Build history of the part. All positions in model axes, mm. A direction names the side the tool comes from. Coordinates: 2 decimals unless noted, no trailing zeros. Write each loop counter-clockwise with the first axis right and the second up, starting at its lowest first coordinate (ties: lowest second). Pieces come first, ordered by that corner, then holes. Notation, with made-up numbers: (15, 19) -> (70, 19) arc R29 ccw to (70, 48) -> close; hole circle Ø10 at (-4.75, -34). An arc over 180 degrees is marked (long way). Write each question's results on one line, items separated by ' | '. Start each with the question number.
Q1. Tool access for faces 1 (the face through (84, 57, 0)), 2 (the face through (-63, -41, 2.9)), 3 (the face through (23, -13, -3)), 4 (the face through (21.48, 18.41, 3.83)): list every direction of +Z, -Z, +X, -X, +Y, -Y with a clear straight run to the whole face (end or side of a thin tool).
Q2. Drop flat-ended pins along their axis: pin 1 Ø13.5 at (x, y) = (89.5, -24) entering from -Z; pin 2 Ø8.5 at (x, y) = (11, 34.5) entering from -Z. Give the stop position or say it passes through.
Q3. Drill centre lines: line 1 (X direction, y = 60, z = -0.5); line 2 (X direction, y = 15, z = 0.5); line 3 (Z direction, x = -38.5, y = -1). Where is each one in solid material? Low to high.
Q4. Saw through at C-C on x = 81. Give the cut face in (y, z), and give its area (3 significant figures).
Q5. Two-plate mould, pull along X, no slides. Class faces 5 (the face through (-37, 45, -3)), 6 (the face through (11.09, 35.17, 3.83)), 7 (the face through (52.7, -27.8, -3)): released by +X, released by -X, zero draft, split by the parting line, or undercut.
Q6. Saw through at A-A on y = -2. Give the cut face in (x, z), and give its area (3 significant figures).
from build123d import *

# Parameters (mm, degrees)
SKETCH_1_W           = 180
SKETCH_1_H           = 108
EXTRUDE_4_DEPTH      = 6
SKETCH_3_R           = 2.85
EXTRUDE_8_DEPTH      = 5.7
SKETCH_4_R           = 2.85
EXTRUDE_9_DEPTH      = 3.1
SKETCH_5_R           = 2.85
CUT_EXTRUDE_1_DEPTH  = 3.1
SKETCH_7_R           = 2.85
CUT_EXTRUDE_2_DEPTH  = 3.1
SKETCH_8_R           = 2.85
CUT_EXTRUDE_3_DEPTH  = 3.1
SKETCH_9_R           = 2.85
CUT_EXTRUDE_4_DEPTH  = 3.1
SKETCH_10_R          = 1.51
CUT_EXTRUDE_5_DEPTH  = 3.1
SKETCH_11_R          = 1.51
CUT_EXTRUDE_6_DEPTH  = 3.1
SKETCH_12_R          = 1.51
CUT_EXTRUDE_7_DEPTH  = 3.1
SKETCH_13_R          = 1.51
CUT_EXTRUDE_8_DEPTH  = 3.1
SKETCH_14_W          = 21
SKETCH_14_H          = 31
CUT_EXTRUDE_10_DEPTH = 10
CUT_EXTRUDE_12_DEPTH = 1
EXTRUDE_10_DEPTH     = 4.4
EXTRUDE_12_DEPTH     = 4.4
SKETCH_18_R          = 3
EXTRUDE_15_DEPTH     = 108
SKETCH_21_R          = 3
EXTRUDE_16_DEPTH     = 180


with BuildPart() as part:
    # 草图1 → 凸台-拉伸4 (new body)
    with BuildSketch(Plane.XY):
        with Locations((22.665747166, 11.024023211)):
            Rectangle(SKETCH_1_W, SKETCH_1_H)
    extrude(amount=EXTRUDE_4_DEPTH)

    # 草图3 → 凸台-拉伸8 (add)
    with BuildSketch(Plane.XY.offset(6)):
        with Locations((109.165747166, 61.524023211)):
            Circle(SKETCH_3_R)
    extrude(amount=-EXTRUDE_8_DEPTH)

    # 草图4 → 凸台-拉伸9 (add)
    with BuildSketch(Plane.XY.offset(6)):
        with Locations((-63.834252834, 61.524023211)):
            Circle(SKETCH_4_R)
    extrude(amount=-EXTRUDE_9_DEPTH)

    # 草图5 → 切除-拉伸1 (cut)
    with BuildSketch(Plane.XY.offset(6)):
        with Locations((-63.834252834, 61.524023211)):
            Circle(SKETCH_5_R)
    extrude(amount=-CUT_EXTRUDE_1_DEPTH, mode=Mode.SUBTRACT)

    # 草图7 → 切除-拉伸2 (cut)
    with BuildSketch(Plane.XY.offset(6)):
        with Locations((109.165747166, 61.524023211)):
            Circle(SKETCH_7_R)
    extrude(amount=-CUT_EXTRUDE_2_DEPTH, mode=Mode.SUBTRACT)

    # 草图8 → 切除-拉伸3 (cut)
    with BuildSketch(Plane.XY.offset(6)):
        with Locations((-63.834252834, -39.475976789)):
            Circle(SKETCH_8_R)
    extrude(amount=-CUT_EXTRUDE_3_DEPTH, mode=Mode.SUBTRACT)

    # 草图9 → 切除-拉伸4 (cut)
    with BuildSketch(Plane.XY.offset(6)):
        with Locations((109.165747166, -39.475976789)):
            Circle(SKETCH_9_R)
    extrude(amount=-CUT_EXTRUDE_4_DEPTH, mode=Mode.SUBTRACT)

    # 草图10 → 切除-拉伸5 (cut)
    with BuildSketch(Plane(origin=(0, 0, 0), x_dir=(-1, 0, 0), z_dir=(0, 0, -1))):
        with Locations((-109.165747166, 61.524023211)):
            Circle(SKETCH_10_R)
    extrude(amount=-CUT_EXTRUDE_5_DEPTH, mode=Mode.SUBTRACT)

    # 草图11 → 切除-拉伸6 (cut)
    with BuildSketch(Plane(origin=(0, 0, 0), x_dir=(-1, 0, 0), z_dir=(0, 0, -1))):
        with Locations((-109.165747166, -39.475976789)):
            Circle(SKETCH_11_R)
    extrude(amount=-CUT_EXTRUDE_6_DEPTH, mode=Mode.SUBTRACT)

    # 草图12 → 切除-拉伸7 (cut)
    with BuildSketch(Plane(origin=(0, 0, 0), x_dir=(-1, 0, 0), z_dir=(0, 0, -1))):
        with Locations((63.834252834, 61.524023211)):
            Circle(SKETCH_12_R)
    extrude(amount=-CUT_EXTRUDE_7_DEPTH, mode=Mode.SUBTRACT)

    # 草图13 → 切除-拉伸8 (cut)
    with BuildSketch(Plane(origin=(0, 0, 0), x_dir=(-1, 0, 0), z_dir=(0, 0, -1))):
        with Locations((63.834252834, -39.475976789)):
            Circle(SKETCH_13_R)
    extrude(amount=-CUT_EXTRUDE_8_DEPTH, mode=Mode.SUBTRACT)

    # 草图14 → 切除-拉伸10 (cut)
    with BuildSketch(Plane.XY.offset(6)):
        with Locations((17.165747166, 24.524023211)):
            Rectangle(SKETCH_14_W, SKETCH_14_H)
    extrude(amount=-CUT_EXTRUDE_10_DEPTH, mode=Mode.SUBTRACT)

    # 草图15 → 切除-拉伸12 (cut)
    with BuildSketch(Plane.XY.offset(6)):
        with BuildLine():
            Line((6.665747166, 42.91898623), (27.665747166, 42.91898623))
            ThreePointArc((27.665747166, 42.91898623), (28.389350728, 42.195382667), (27.665747166, 41.471779105))
            Line((27.665747166, 41.471779105), (6.665747166, 41.471779105))
            ThreePointArc((6.665747166, 41.471779105), (5.942143603, 42.195382667), (6.665747166, 42.91898623))
        make_face()
    extrude(amount=-CUT_EXTRUDE_12_DEPTH, mode=Mode.SUBTRACT)

    # 草图16 → 凸台-拉伸10 (add)
    with BuildSketch(Plane.XY.offset(6)):
        with BuildLine():
            Line((28.493665856, 39.463175066), (7.493665856, 8.463175066))
            ThreePointArc((7.493665856, 8.463175066), (6.104899021, 8.19610452), (5.837828475, 9.584871356))
            Line((5.837828475, 9.584871356), (26.837828475, 40.584871356))
            ThreePointArc((26.837828475, 40.584871356), (28.226595311, 40.851941901), (28.493665856, 39.463175066))
        make_face()
        with BuildLine():
            Line((24.870121619, 39.463175066), (7.493665856, 13.812216559))
            ThreePointArc((7.493665856, 13.812216559), (6.104899021, 13.545146014), (5.837828475, 14.933912849))
            Line((5.837828475, 14.933912849), (23.214284238, 40.584871356))
            ThreePointArc((23.214284238, 40.584871356), (24.603051073, 40.851941901), (24.870121619, 39.463175066))
        make_face()
        with BuildLine():
            Line((21.246577381, 39.463175066), (7.493665856, 19.161258052))
            ThreePointArc((7.493665856, 19.161258052), (6.104899021, 18.894187507), (5.837828475, 20.282954343))
            Line((5.837828475, 20.282954343), (19.59074, 40.584871356))
            ThreePointArc((19.59074, 40.584871356), (20.979506836, 40.851941901), (21.246577381, 39.463175066))
        make_face()
        with BuildLine():
            Line((17.623033144, 39.463175066), (7.493665856, 24.510299546))
            ThreePointArc((7.493665856, 24.510299546), (6.104899021, 24.243229001), (5.837828475, 25.631995836))
            Line((5.837828475, 25.631995836), (15.967195763, 40.584871356))
            ThreePointArc((15.967195763, 40.584871356), (17.355962599, 40.851941901), (17.623033144, 39.463175066))
        make_face()
        with BuildLine():
            Line((13.975285013, 39.427445509), (7.493665856, 29.859341039))
            ThreePointArc((7.493665856, 29.859341039), (6.104899021, 29.592270494), (5.837828475, 30.98103733))
            Line((5.837828475, 30.98103733), (12.319447632, 40.549141799))
            ThreePointArc((12.319447632, 40.549141799), (13.708214468, 40.816212345), (13.975285013, 39.427445509))
        make_face()
        with BuildLine():
            Line((10.375944669, 39.463175066), (7.493665856, 35.208382533))
            ThreePointArc((7.493665856, 35.208382533), (6.104899021, 34.941311987), (5.837828475, 36.330078823))
            Line((5.837828475, 36.330078823), (8.720107288, 40.584871356))
            ThreePointArc((8.720107288, 40.584871356), (10.108874124, 40.851941901), (10.375944669, 39.463175066))
        make_face()
        with BuildLine():
            Line((28.493665856, 34.114133572), (11.117210094, 8.463175066))
            ThreePointArc((11.117210094, 8.463175066), (9.728443258, 8.19610452), (9.461372713, 9.584871356))
            Line((9.461372713, 9.584871356), (26.837828475, 35.235829863))
            ThreePointArc((26.837828475, 35.235829863), (28.226595311, 35.502900408), (28.493665856, 34.114133572))
        make_face()
        with BuildLine():
            Line((28.493665856, 28.765092079), (14.740754331, 8.463175066))
            ThreePointArc((14.740754331, 8.463175066), (13.351987496, 8.19610452), (13.08491695, 9.584871356))
            Line((13.08491695, 9.584871356), (26.837828475, 29.886788369))
            ThreePointArc((26.837828475, 29.886788369), (28.226595311, 30.153858915), (28.493665856, 28.765092079))
        make_face()
        with BuildLine():
            Line((28.493665856, 18.067009092), (21.839365483, 8.243994256))
            ThreePointArc((21.839365483, 8.243994256), (20.450598648, 7.976923711), (20.183528102, 9.365690546))
            Line((20.183528102, 9.365690546), (26.837828475, 19.188705383))
            ThreePointArc((26.837828475, 19.188705383), (28.226595311, 19.455775928), (28.493665856, 18.067009092))
        make_face()
        with BuildLine():
            Line((28.493665856, 12.717967599), (25.611387044, 8.463175066))
            ThreePointArc((25.611387044, 8.463175066), (24.222620208, 8.19610452), (23.955549663, 9.584871356))
            Line((23.955549663, 9.584871356), (26.837828475, 13.839663889))
            ThreePointArc((26.837828475, 13.839663889), (28.226595311, 14.106734434), (28.493665856, 12.717967599))
        make_face()
        with BuildLine():
            Line((28.493665856, 23.416050586), (18.364298569, 8.463175066))
            ThreePointArc((18.364298569, 8.463175066), (16.975531733, 8.19610452), (16.708461188, 9.584871356))
            Line((16.708461188, 9.584871356), (26.837828475, 24.537746876))
            ThreePointArc((26.837828475, 24.537746876), (28.226595311, 24.804817421), (28.493665856, 23.416050586))
        make_face()
    extrude(amount=-EXTRUDE_10_DEPTH)

    # 草图17 → 凸台-拉伸12 (add)
    with BuildSketch(Plane.XY.offset(6)):
        Polygon((9.291077122, 41.427731587), (10.946914503, 40.306035296), (9.559645246, 38.258161632), (7.903807865, 39.379857922), align=None)
        Polygon((13.049495166, 41.419687565), (14.652090321, 40.219395608), (13.183189483, 38.258161632), (11.580594328, 39.458453588), align=None)
        Polygon((16.598688708, 41.312908479), (18.201283863, 40.112616523), (16.753491495, 38.179565965), (15.15089634, 39.379857922), align=None)
        Polygon((23.799395039, 41.251005631), (25.404854584, 40.05494206), (23.929168948, 38.074149695), (22.323709403, 39.270213267), align=None)
        Polygon((20.294085137, 41.416455751), (21.899544682, 40.220392179), (20.356002546, 38.148516976), (18.750543001, 39.344580548), align=None)
        Polygon((27.059349697, 31.996809719), (29.592825756, 35.991789111), (27.903049923, 37.063385782), (25.369573865, 33.06840639), align=None)
        Polygon((27.059349697, 26.647768225), (29.657516879, 30.835687648), (27.956643474, 31.890902187), (25.358476292, 27.702982765), align=None)
        Polygon((27.059349697, 21.298726732), (29.809729018, 25.762891731), (28.105364864, 26.812953261), (25.354985543, 22.348788261), align=None)
        Polygon((27.059349697, 15.949685239), (29.875638884, 20.653316626), (28.157020256, 21.682335837), (25.340731069, 16.97870445), align=None)
        Polygon((27.400761437, 11.104632504), (30.093714703, 15.079944467), (28.437877322, 16.201640757), (25.744924056, 12.226328794), align=None)
        Polygon((24.34904045, 6.839114616), (22.743580905, 8.035178188), (24.531450984, 10.435011402), (26.136910529, 9.23894783), align=None)
        Polygon((20.616325121, 6.692575775), (19.010865576, 7.888639346), (20.907906746, 10.435011402), (22.513366292, 9.23894783), align=None)
        Polygon((17.217009332, 6.999947538), (15.611549786, 8.196011109), (17.33210575, 10.505489519), (18.937565295, 9.309425947), align=None)
        Polygon((13.752364906, 7.191393443), (12.14690536, 8.387457015), (13.545436794, 10.264686364), (15.15089634, 9.068622793), align=None)
        Polygon((10.142404174, 7.231469503), (8.536944628, 8.427533074), (10.085017275, 10.505489519), (11.69047682, 9.309425947), align=None)
        Polygon((7.407914057, 17.251658231), (4.395376532, 12.804579029), (6.051213913, 11.682882738), (9.063751438, 16.129961941), align=None)
        Polygon((7.235662462, 22.346423561), (4.352783087, 18.090744484), (6.008620468, 16.969048193), (8.891499842, 21.22472727), align=None)
        Polygon((7.235662462, 27.695465054), (5.052244478, 24.472324221), (6.708081859, 23.35062793), (8.891499842, 26.573768764), align=None)
        Polygon((7.235662462, 33.044506547), (4.876433622, 29.202971295), (6.582399671, 28.155274467), (8.94162851, 31.996809719), align=None)
        Polygon((6.83097858, 37.796157549), (8.536944628, 36.74846072), (6.3595402, 33.202990382), (4.653574152, 34.250687211), align=None)
    extrude(amount=-EXTRUDE_12_DEPTH)

    # 草图18 → 凸台-拉伸15 (add)
    with BuildSketch(Plane(origin=(0, 65.024023211, 0), x_dir=(1, 0, 0), z_dir=(0, 1, 0))):
        with Locations((-7.334252834, 0)):
            Circle(SKETCH_18_R)
        with Locations((52.665747166, 0)):
            Circle(SKETCH_18_R)
    extrude(amount=-EXTRUDE_15_DEPTH)

    # 草图21 → 凸台-拉伸16 (add)
    with BuildSketch(Plane(origin=(112.665747166, 0, 0), x_dir=(0, 0, -1), z_dir=(1, 0, 0))):
        with Locations((0, -12.975976789)):
            Circle(SKETCH_21_R)
        with Locations((0, 45.024023211)):
            Circle(SKETCH_21_R)
    extrude(amount=-EXTRUDE_16_DEPTH)


solid = part.part
Returned:
1) face 1: -Z, +X, +Y | face 2: +Z | face 3: -Z | face 4: +Z, -Z
2) pin 1: stops at z = 0 | pin 2: stops at z = 1.6
3) line 1: x = -10.29 to -4.38, 49.71 to 55.62 | line 2: x = -67.33 to 6.67, 27.67 to 112.67 | line 3: z = 0 to 6
4) outline: (-42.98, 0) -> (-15.98, 0) arc R3 ccw to (-9.98, 0) -> (42.02, 0) arc R3 ccw to (48.02, 0) -> (65.02, 0) -> (65.02, 6) -> (-42.98, 6) -> close | area: 676 mm2
5) face 5: zero draft | face 6: undercut | face 7: undercut
6) outline: (-67.33, 0) -> (-10.33, 0) arc R3 ccw to (-4.33, 0) -> (49.67, 0) arc R3 ccw to (55.67, 0) -> (112.67, 0) -> (112.67, 6) -> (-67.33, 6) -> close | area: 1,110 mm2
